from build123d import *

# Parameters (mm, degrees)
F0_W     = 63.5
F0_H     = 63.5
F1_DEPTH = 31.75
F2_SIZE2 = 63.49999
F2_SIZE  = 20.31999
F4_DEPTH = 114.3


# Not quite as in the source:
# - a fillet or chamfer is up to 0.001 mm smaller than in the source, because OpenCascade refuses the exact size


with BuildPart() as f1:
    # F0 (on Right) → F1 (new body, symmetric)
    with BuildSketch(Plane.YZ):
        Rectangle(F0_W, F0_H)
    extrude(amount=F1_DEPTH, both=True)

    # F2 (size 20.32 and 63.5 in the source; OpenCascade refuses exactly that, so slightly less here)
    f2_edges = [f1.edges().sort_by_distance(p)[0] for p in [
        (31.75, -31.75, 0),
        (31.75, 0, 31.75),
        (31.75, 31.75, 0),
        (31.75, 0, -31.75),
    ]]
    f2_side = f1.faces().sort_by_distance((31.75, 0, 0))[0]
    chamfer(f2_edges, length=F2_SIZE, length2=F2_SIZE2, reference=f2_side)

    # F3 (on face) → F4 (join)
    with BuildSketch(Plane(origin=(-31.75, 0, 0), x_dir=(0, -1, 0), z_dir=(-1, 0, 0))):
        Polygon((-31.75, -31.75), (31.75, -31.75), (11.43, -11.43), (-11.43, -11.43), align=None)
    extrude(amount=-F4_DEPTH)


solid = f1.part
Geometry check sheet. Reference: the model listing, model coordinates, mm. A direction names the side the tool comes from. Give positions to 0.01 mm unless a question says otherwise; leave off trailing zeros. Order: outer loops, then holes, each group sorted by start corner. A loop starts at its lowest first (then second) coordinate and runs counter-clockwise, first axis right, second up.
1. Sectioned sample at D-D (x = 19). Record the boundary of the cut face in (y, z).
Completed:
outline: (-31.75, -31.75) - (31.75, -31.75) - (15.51, -15.51) - (15.51, 15.51) - (-15.51, 15.51) - (-15.51, -15.51) - close
2. Sectioned sample at B-B (x = -6.5). Record the boundary of the cut face in (y, z), then the cut area to 3 significant figures.
Completed:
outline: (-31.75, -31.75) - (31.75, -31.75) - (23.67, -23.67) - (23.67, 23.67) - (-23.67, 23.67) - (-23.67, -23.67) - close
area: 2,690 mm2
3. Scan lines: line 1 (Z direction, x = 70.5, y = -1); line 2 (X direction, y = 6, z = -0.5); line 3 (Z direction, x = 23, y = -14). Record each from-to range of solid material in increasing order.
Completed:
line 1: z = -31.75 to -11.43
line 2: x = -31.75 to 31.75
line 3: z = -31.75 to 14.23
4. Access from +Z, -Z, +X, -X, +Y, -Y to the whole of each face (thin tool, end or side, straight path). Record for faces 1 (the face through (57, 0, -11.43)), 2 (the face through (-7.5, -23.99, -0.44)), 3 (the face through (-7.5, 23.99, -0.44)).
Completed:
face 1: +Z, +X, +Y, -Y
face 2: +Z, +X, -Y
face 3: +Z, +X, +Y
5. Depth check by flat-ended pin: pin 1 (4 mm diameter, centred on x = 66.5, z = -22.5, fed in from +Y); pin 2 (3 mm diameter, centred on x = 45, y = 17.5, fed in from +Z); pin 3 (4 mm diameter, centred on x = 18.5, z = -20, fed in from -Y). Enter the tip coordinate at first touch or a pass-through.
Completed:
pin 1: stops at y = 24.5
pin 2: stops at z = -16
pin 3: stops at y = -22
